Geometry: see drawing. Coordinates: mm, zero at the bounding-box minimum. A direction names the side the tool comes from. Coordinates: 2 decimals unless noted, no trailing zeros. Loops run counter-clockwise (first coordinate to the right, second up) from the corner with the lowest first, then second, coordinate; pieces in that order, holes last.
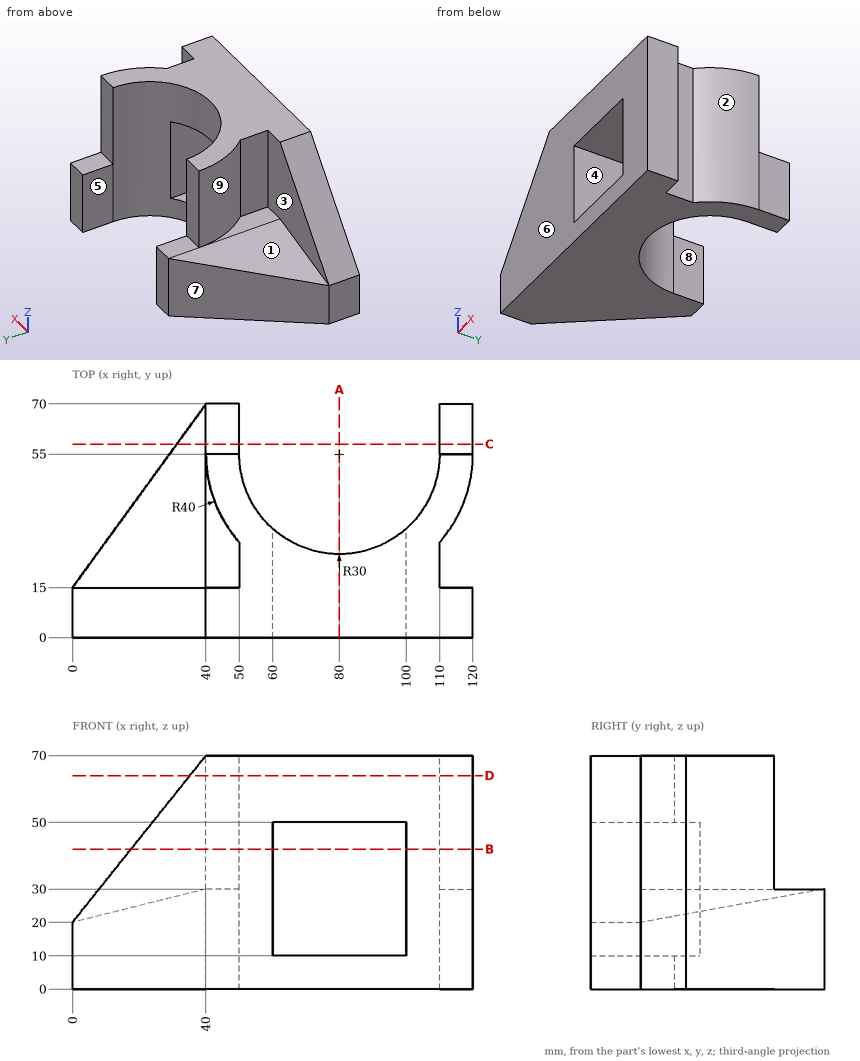
Item 1: Section query C-C (y = 58). Output: boundary loops of the cut face in (x, z).
Result:
outline: (31.27, 0) - (50, 0) - (50, 30) - (40, 30) - (31.27, 27.82) - close; (110, 0) - (120, 0) - (120, 30) - (110, 30) - close
Item 2: Section query A-A (x = 80). Output: boundary loops of the cut face in (y, z).
Result:
outline: (0, 0) - (25, 0) - (25, 10) - (0, 10) - close; (0, 50) - (25, 50) - (25, 70) - (0, 70) - close
Item 3: Section query D-D (z = 64). Output: boundary loops of the cut face in (x, y).
Result:
outline: (35.2, 0) - (120, 0) - (120, 15) - (110, 15) - (110, 28.54) arc R40 ccw to (120, 55) - (110, 55) arc R30 cw to (50, 55) - (40, 55) arc R40 ccw to (50, 28.54) - (50, 15) - (35.2, 15) - close
Item 4: Contact query for flat-ended pins moving along their axis: P1, Ø5, axis at x = 44.5, y = 59, coming from the +Z side; P2, Ø11, axis at y = 21.5, z = 49, coming from the +X side; P3, Ø8, axis at y = 43, z = 61, coming from the -X side. Output: stop coordinate, or through.
Result:
P1: stops at z = 30
P2: stops at x = 110
P3: stops at x = 40.81
Item 5: Reachability of the marked faces 1, 2, 3, 4 and 5 from +Z, -Z, +X, -X, +Y, -Y: full face, straight path, thin tool, end or side. Return the list, or none.
Result:
face 1: +Z, -X, +Y
face 2: +Z, -Z, +X
face 3: +Z, -X
face 4: +Y, -Y
face 5: +Z, -Z, +Y
Item 6: Section query B-B (z = 42). Output: boundary loops of the cut face in (x, y).
Result:
outline: (17.6, 0) - (60, 0) - (60, 32.64) arc R30 cw to (50, 55) - (40, 55) arc R40 ccw to (50, 28.54) - (50, 15) - (17.6, 15) - close; (100, 0) - (120, 0) - (120, 15) - (110, 15) - (110, 28.54) arc R40 ccw to (120, 55) - (110, 55) arc R30 cw to (100, 32.64) - close
Item 7: Line query: L1, parallel to X at y = 27, z = 42.5; L2, parallel to Y at x = 15.5, z = 37; L3, parallel to X at y = 44.5, z = 12.5. Output: solid intervals per line, ascending.
Result:
L1: x = 50 to 60, 100 to 110
L2: y = 0 to 15
L3: x = 21.45 to 51.9, 108.1 to 118.6
Item 8: Mould query, pull axis Y, two halves, no side actions, for the marked faces 6, 7, 8 and 9. Classes: +Y half, -Y half, draft (parallel to the pull), parting line (faces both ways), or undercut.
Result:
face 6: -Y half
face 7: +Y half
face 8: draft
face 9: undercut
